Work out the finished part from the listing and answer in its coordinate system (mm). A direction names the side the tool comes from. Give positions to 0.01 mm unless a question says otherwise; leave off trailing zeros. Order: outer loops, then holes, each group sorted by start corner. A loop starts at its lowest first (then second) coordinate and runs counter-clockwise, first axis right, second up. Notation, with made-up numbers: (29, 60.5) - (88, 60.5) arc R12 cw to (88, 67.5) - close; hole circle Ø3 at (-5, 85.5). An arc over 180 degrees is marked (long way). Put each result on its own line as item: value.
```python
from build123d import *

# Parameters (mm, degrees)
OUTER_SKETCH_R                = 10.25
OUTER_DEPTH                   = 2
INNER_SKETCH_R                = 7.25
INNER_DEPTH                   = 3
ODEBRAT_VYSUNUT_M2_DEPTH      = 15.746272134
ODEBRAT_VYSUNUT_M2_DEPTH_BACK = 15.746272134
SKICA8_R                      = 2.5


with BuildPart() as part:
    # Outer sketch → Outer (new body)
    with BuildSketch(Plane.XY):
        Circle(OUTER_SKETCH_R)
    extrude(amount=OUTER_DEPTH)

    # Inner sketch → Inner (add)
    with BuildSketch(Plane.XY.offset(2)):
        Circle(INNER_SKETCH_R)
    extrude(amount=INNER_DEPTH)

    # Skica8 → Odebrat vysunutím2 (cut, two sides: drawn at the far end of the back side and taken through both)
    with BuildSketch(Plane(origin=(0, -0.042117416, 2.457882584), x_dir=(1, 0, 0), z_dir=(0, -0.7071067811865476, 0.7071067811865476)).offset(-ODEBRAT_VYSUNUT_M2_DEPTH_BACK)):
        with Locations(Location((-3, 0.413116411, 0), (0, 0, 270))):
            Circle(SKICA8_R)
        with Locations(Location((3, 0.413116411, 0), (0, 0, 270))):
            Circle(SKICA8_R)
    extrude(amount=ODEBRAT_VYSUNUT_M2_DEPTH + ODEBRAT_VYSUNUT_M2_DEPTH_BACK, mode=Mode.SUBTRACT)


solid = part.part
```
(1) Section D-D, the plane x = 4.25 is taken. Write down the section's boundary in (y, z), then the cut area to 3 significant figures.
Geometry check:
outline: (-9.33, 0) - (-0.06, 0) - (-5.06, 5) - (-5.87, 5) - (-5.87, 2) - (-9.33, 2) - close; (1.06, 5) - (6.06, 0) - (9.33, 0) - (9.33, 2) - (5.87, 2) - (5.87, 5) - close
area: 41.9 mm²
(2) Straight lines are drawn through the part: line 1 (X direction, y = 1, z = 4.45); line 2 (X direction, y = -2.75, z = 3.85); line 3 (Z direction, x = 1, y = 8). For each, find the intervals that lie inside material, in ascending order.
Geometry check:
line 1: x = -7.18 to -4.8, -1.2 to 1.2, 4.8 to 7.18
line 2: x = -6.71 to -5.11, -0.89 to 0.89, 5.11 to 6.71
line 3: z = 0 to 2
(3) Section A-A, the plane x = -2.5 is taken. Write down the section's boundary in (y, z).
Geometry check:
outline: (-9.94, 0) - (-0.46, 0) - (-5.46, 5) - (-6.81, 5) - (-6.81, 2) - (-9.94, 2) - close; (1.46, 5) - (6.46, 0) - (9.94, 0) - (9.94, 2) - (6.81, 2) - (6.81, 5) - close
(4) A tool of negligible diameter and unlimited length cuts with its end or side. For faces 5 (the face through (-2.222, -10.006, 0.986)), 6 (the face through (-2.4, 7, 2)), from which of +Z, -Z, +X, -X, +Y, -Y can it reach the whole face along a straight path? Write none if from no direction.
Geometry check:
face 5: +Z, -Z
face 6: +Z
(5) Determine the mould class of faces 1 (the face through (3.35, -6.43, 3.48)), 2 (the face through (-2.89, 2.36, 4.17)), 3 (the face through (5.48, 0.83, 2.63)), 4 (the face through (0, 0, 0)) for opening direction Y: pulls with the +Y half, pulls with the -Y half, needs draft (parallel to the pull), parting line crosses it, or undercut.
Geometry check:
face 1: parting line crosses it
face 2: undercut
face 3: undercut
face 4: needs draft
(6) Section C-C, the plane y = -6.25 is taken. Write down the section's boundary in (x, z), then the cut area to 3 significant figures.
Geometry check:
outline: (-8.12, 0) - (8.12, 0) - (8.12, 2) - (3.67, 2) - (3.67, 5) - (-3.67, 5) - (-3.67, 2) - (-8.12, 2) - close
area: 54.5 mm²
(7) Section B-B, the plane x = 0 is taken. Write down the section's boundary in (y, z), then the cut area to 3 significant figures.
Geometry check:
outline: (-10.25, 0) - (10.25, 0) - (10.25, 2) - (7.25, 2) - (7.25, 5) - (-7.25, 5) - (-7.25, 2) - (-10.25, 2) - close
area: 84.5 mm²
(8) Given pin 1 (2 mm diameter, centred on y = 1, z = 4, fed in from +X); pin 2 (8 mm diameter, centred on x = -7, y = -3.5, fed in from +Z); pin 3 (1 mm diameter, centred on x = -6, z = 0.5, fed in from -Y); pin 4 (1.5 mm diameter, centred on y = 3.5, z = 2, fed in from +X), each flat-ended and moving along its own axis, determine where each tip first touches the part or whether it passes through.
Geometry check:
pin 1: stops at x = 7.25
pin 2: stops at z = 5
pin 3: stops at y = -8.65
pin 4: stops at x = 9.87
